Geometry: see drawing. Coordinates: mm, zero at the bounding-box minimum. A direction names the side the tool comes from. Give positions to 0.01 mm unless a question says otherwise; leave off trailing zeros. Order: outer loops, then holes, each group sorted by start corner. A loop starts at its lowest first (then second) coordinate and runs counter-clockwise, first axis right, second up. Notation, with made-up numbers: (70.25, 86.25) - (78.25, 86.25) arc R22 cw to (78.25, 92.25) - close; hole circle Ø3 at (50, 40). An arc over 180 degrees is marked (long way). One line per item, written item: value. Start each with the question number.
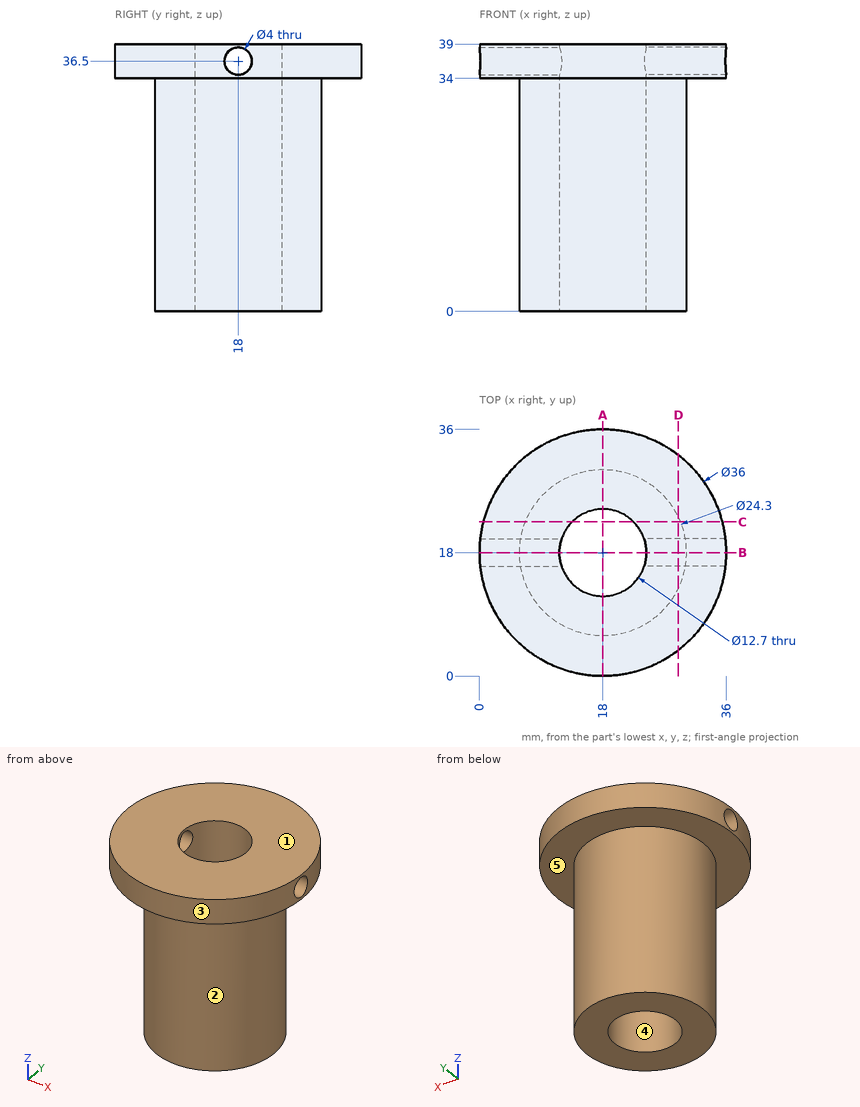
1. Section A-A on x = 18. Return the cut outline in (y, z), then the cut area to 3 significant figures.
2. Section D-D on x = 29. Return the cut outline in (y, z), then the cut area to 3 significant figures.
3. Set-up query: the marked faces 1 and 2. Return all of +Z, -Z, +X, -X, +Y, -Y with unobstructed straight access to the full face (end or side cutting, diameter ignored); none if empty.
4. Section B-B on y = 18. Return the cut outline in (x, z), then the cut area to 3 significant figures.
5. Contact query for flat-ended pins moving along their axis: pin 1 Ø1 at (x, z) = (24, 10.5) entering from -Y; pin 2 Ø4 at (y, z) = (28, 25) entering from +X; pin 3 Ø12 at (x, z) = (10, 31) entering from -Y; pin 4 Ø3 at (y, z) = (18, 36.5) entering from -X. Output: stop coordinate, or through.
6. Ray query, L1, parallel to Y at x = 18, z = 24.5; L2, parallel to Z at x = 2.5, y = 17; L3, parallel to Y at x = 21, z = 14. Return the intervals inside material, ascending.
7. Draft query along X for the marked faces 3, 4 and 5. Return one class per face: pulls with the +X half, pulls with the -X half, needs draft (parallel to the pull), parting line crosses it, or undercut.
8. Section C-C on y = 22.5. Return the cut outline in (x, z).
Data:
1. outline: (0, 34) - (5.85, 34) - (5.85, 0) - (11.65, 0) - (11.65, 39) - (0, 39) - close; (24.35, 0) - (30.15, 0) - (30.15, 34) - (36, 34) - (36, 39) - (24.35, 39) - close
1. area: 511 mm2
2. outline: (3.75, 34) - (12.84, 34) - (12.84, 0) - (23.16, 0) - (23.16, 34) - (32.25, 34) - (32.25, 39) - (3.75, 39) - close; hole circle Ø4 at (18, 36.5)
2. area: 481 mm2
3. face 1: +Z, +X, -X, +Y, -Y
3. face 2: -Z
4. outline: (0, 34) - (5.85, 34) - (5.85, 0) - (11.65, 0) - (11.65, 34.5) - (0, 34.5) - close; (0, 38.5) - (11.65, 38.5) - (11.65, 39) - (0, 39) - close; (24.35, 0) - (30.15, 0) - (30.15, 34) - (36, 34) - (36, 34.5) - (24.35, 34.5) - close; (24.35, 38.5) - (36, 38.5) - (36, 39) - (24.35, 39) - close
4. area: 418 mm2
5. pin 1: stops at y = 7.17
5. pin 2: stops at x = 27.14
5. pin 3: stops at y = 0.22
5. pin 4: passes through
6. L1: y = 5.85 to 11.65, 24.35 to 30.15
6. L2: z = 34 to 34.77, 38.23 to 39
6. L3: y = 6.23 to 12.4, 23.6 to 29.77
7. face 3: parting line crosses it
7. face 4: undercut
7. face 5: needs draft
8. outline: (0.57, 34) - (6.71, 34) - (6.71, 0) - (13.52, 0) - (13.52, 39) - (0.57, 39) - close; (22.48, 0) - (29.29, 0) - (29.29, 34) - (35.43, 34) - (35.43, 39) - (22.48, 39) - close
